```python
from build123d import *

# Parameters (mm, degrees)
SKETCH1_R              = 28
BOSS_EXTRUDE1_DEPTH    = 10
SKETCH2_R              = 10
BOSS_EXTRUDE2_DEPTH    = 22
SKETCH4_R              = 4
CUT_EXTRUDE2_DEPTH     = 51.911688245
CHAMFER2_SIZE          = 1
M4_TAPPED_HOLE1_REACH  = 54.077
M4_TAPPED_HOLE1_BORE_R = 1.65
CIRPATTERN2_COUNT      = 2
CIRPATTERN2_ANGLE      = 90


with BuildPart() as part:
    # Sketch1 → Boss-Extrude1 (new body)
    with BuildSketch(Plane.XY):
        Circle(SKETCH1_R)
    extrude(amount=BOSS_EXTRUDE1_DEPTH)

    # Sketch2 → Boss-Extrude2 (add)
    with BuildSketch(Plane.XY.offset(10)):
        Circle(SKETCH2_R)
    extrude(amount=BOSS_EXTRUDE2_DEPTH)

    # Sketch4 → Cut-Extrude2 (cut, through all)
    with BuildSketch(Plane.XY.offset(32)):
        Circle(SKETCH4_R)
    extrude(amount=-CUT_EXTRUDE2_DEPTH, mode=Mode.SUBTRACT)

    # Chamfer2
    chamfer2_edges = [part.edges().sort_by_distance(p)[0] for p in [
        (-4, 0, 32),
        (-10, 0, 10),
        (-10, 0, 32),
    ]]
    chamfer(chamfer2_edges, length=CHAMFER2_SIZE)

    # M4 Tapped Hole1 bore (on position points) → M4 Tapped Hole1 (cut, up to next)
    with BuildSketch(Plane(origin=(0, 10, 22), x_dir=(1, 0, 0), z_dir=(0, 1, 0)), mode=Mode.PRIVATE) as m4_tapped_hole1_sk1:
        Circle(M4_TAPPED_HOLE1_BORE_R)
    m4_tapped_hole1_tool1 = extrude(m4_tapped_hole1_sk1.sketch, amount=-M4_TAPPED_HOLE1_REACH, mode=Mode.PRIVATE) & part.part
    m4_tapped_hole1 = m4_tapped_hole1_tool1.solids().sort_by_distance((0, 10, 22))[0]
    add(m4_tapped_hole1, mode=Mode.SUBTRACT)

    # CirPattern2: M4 Tapped Hole1 ×2 about axis
    cirpattern2_axis = Axis((0, 0, 32), (0, 0, -1))
    for i in range(1, CIRPATTERN2_COUNT):
        add(m4_tapped_hole1.rotate(cirpattern2_axis, i * CIRPATTERN2_ANGLE / (CIRPATTERN2_COUNT - 1)), mode=Mode.SUBTRACT)


solid = part.part
```
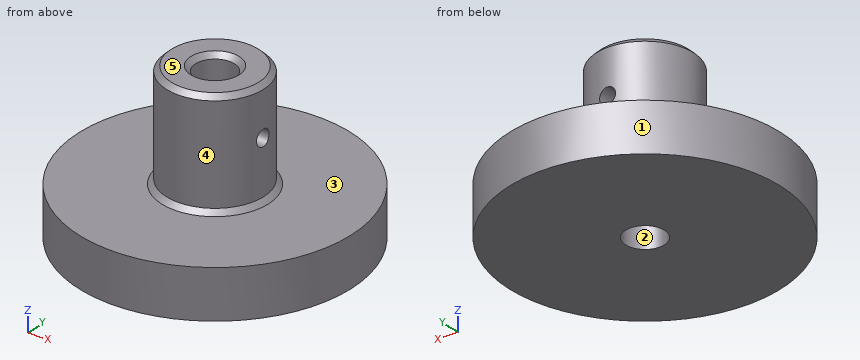
Here's how the part is built. I have some questions about the finished solid (model axes, mm). Face numbers are marked on the shaded views. A direction names the side the tool comes from. Coordinates: 2 decimals unless noted, no trailing zeros. Write each loop counter-clockwise with the first axis right and the second up, starting at its lowest first coordinate (ties: lowest second). Pieces come first, ordered by that corner, then holes. Notation, with made-up numbers: (10, 53.25) -> (25, 53.25) arc R31 ccw to (25, 83.25) -> close; hole circle Ø5 at (39, 89.5). An arc over 180 degrees is marked (long way). Use a Markdown table: item, result. Add a question column.
(1) For the marked faces 4 and 5, which set-ups out of +Z, -Z, +X, -X, +Y, -Y let a thin tool reach every point of the face, with its end or its side?
(2) We'd pull the mould along Y, two halves only. Please class the marked faces 1, 2 and 3: +Y half, -Y half, draft (parallel to the pull), parting line (faces both ways), or undercut.
(3) If we section it at C-C, the plane z = 22: Write out the boundary of the cut face in (x, y).
(4) Please list where these lines run through material, in increasing order: line 1 (Z direction, x = -16, y = -8); line 2 (X direction, y = 4, z = 23); line 3 (Y direction, x = 3.5, z = 26).
(5) If we section it at D-D, the plane z = 28.5: Write out the boundary of the cut face in (x, y).
(6) If we section it at A-A, the plane x = 0: Write out the boundary of the cut face in (y, z), and give its area (3 significant figures).
(7) I'm going to push flat-ended pins straight in: P1, Ø2.5, axis at x = 0, z = 22, coming from the +Y side; P2, Ø5.5, axis at y = 0, z = 22, coming from the +X side; P3, Ø8, axis at y = 13, z = 12, coming from the +X side; P4, Ø2, axis at x = 22.5, y = 19.5, coming from the -Z side. Where does each tip first touch, or does it pass through?
Outcome:
| question | item | result |
|---|---|---|
| 1 | face 4 | +Z |
| 1 | face 5 | +Z, +X, -X, +Y, -Y |
| 2 | face 1 | parting line |
| 2 | face 2 | undercut |
| 2 | face 3 | draft |
| 3 | outline | (-1.65, 3.64) -> (-1.65, 9.86) arc R10 ccw (long way) to (9.86, -1.65) -> (3.64, -1.65) arc R4 cw (long way) to start; (1.65, 3.64) arc R4 cw to (3.64, 1.65) -> (9.86, 1.65) arc R10 ccw to (1.65, 9.86) -> close |
| 4 | line 1 | z = 0 to 10 |
| 4 | line 2 | x = -9.17 to -1.31, 1.31 to 9.17 |
| 4 | line 3 | y = -9.37 to -1.94, 1.94 to 9.37 |
| 5 | outline | circle Ø20 at (0, 0); hole circle Ø8 at (0, 0) |
| 6 | outline | (-28, 0) -> (-4, 0) -> (-4, 31) -> (-5, 32) -> (-9, 32) -> (-10, 31) -> (-10, 11) -> (-11, 10) -> (-28, 10) -> close; (4, 0) -> (28, 0) -> (28, 10) -> (11, 10) -> (10, 11) -> (10, 20.35) -> (4, 20.35) -> close; (4, 23.65) -> (10, 23.65) -> (10, 31) -> (9, 32) -> (5, 32) -> (4, 31) -> close |
| 6 | area | 723 mm^2 |
| 7 | P1 | stops at y = -3.8 |
| 7 | P2 | stops at x = 10 |
| 7 | P3 | stops at x = 26.33 |
| 7 | P4 | passes through |
